Autodesk Fusion 360 part; units mm, degrees
sketch "Sketch1" plane through (0, 0, 0) normal (0, 1, 0) x (1, 0, 0)
  line L0 (0, 0) -> (82.5, 0)
  line L1 (82.5, 0) -> (82.5, -70)
  line L2 (82.5, -70) -> (0, -70)
  line L3 (0, -70) -> (0, 0)
  line L4 (2.54, -70) -> (2.54, -48.5)
  line L5 (2.54, -48.5) -> (0, -46.5)
  line L6 (2.54, 0) -> (2.54, -11.5)
  line L7 (2.54, -11.5) -> (0, -13.5)
  dimension "d1" = 82.5
  dimension "d2" = 70
  dimension "d3" = 33
  dimension "d4" = 11.5
  dimension "d5" = 2.54
  dimension "d6" = 2.54
  dimension "d7" = 21.5
  dimension "d8" = 2
extrude "Extrude1" add sketch "Sketch1" along normal blind 2 contours L0 L1 L2 L3 L4 L5 L6 L7
sketch "Sketch2" plane through (0, 2, 0) normal (0, 1, 0) x (-1, 0, 0)
  line L0 (-2.54, 0) -> (-2.54, 11.5)
  line L1 (-2.54, 11.5) -> (0, 13.5)
  line L2 (0, 13.5) -> (0, 46.5)
  line L3 (0, 46.5) -> (-2.54, 48.5)
  line L4 (-2.54, 48.5) -> (-2.54, 70)
  line L5 (-2.54, 70) -> (-82.5, 70)
  line L6 (-82.5, 70) -> (-82.5, 0)
  line L7 (-82.5, 0) -> (-2.54, 0)
  circle A0 centre (-2.54, 44.5) radius 1.6
  circle A1 centre (-54.14, 59.13) radius 1.6
  circle A2 centre (-55.54, 10.87) radius 1.6
  dimension "d11" = 3.2
  dimension "d12" = 2.54
  dimension "d13" = 33
  dimension "d14" = 3.2
  dimension "d15" = 3.2
  dimension "d17" = 10.87
  dimension "d20" = 53
  dimension "d21" = 51.6
  dimension "d22" = 48.26
extrude "Extrude2" cut sketch "Sketch2" against normal blind 2 contours A0 | A1 | A2
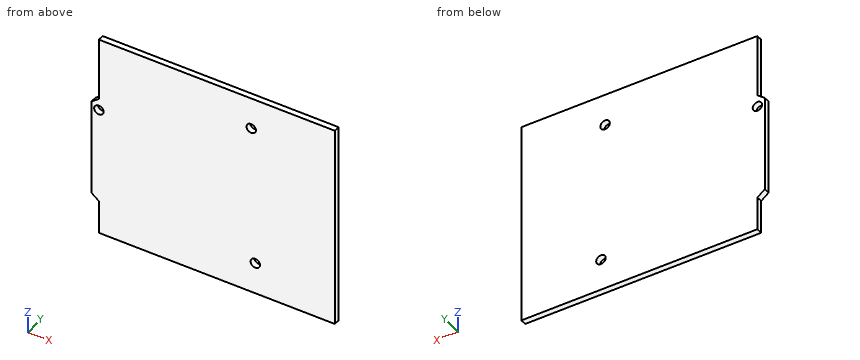
Check sheet for the modelled part. Datum: model origin and axes. Units: mm. Coordinates: 2 decimals unless noted, no trailing zeros. Order: outer loops, then holes, each group sorted by start corner. A loop starts at its lowest first (then second) coordinate and runs counter-clockwise, first axis right, second up. Notation, with made-up numbers: (78, 85.25) -> (135, 85.25) arc R24 ccw to (135, 124.25) -> close; hole circle Ø7 at (59, -10.75). An arc over 180 degrees is marked (long way). Write each question's results on one line, items separated by ' | '. Start each with the question number.
1) Material ranges on line 1 along Z through (x, y) = (55.54, 1.05); line 2 along Z through (x, y) = (54.14, 1); line 3 along X through (y, z) = (1.75, 55), recorded low to high.
2) Depth check by flat-ended pin: pin 1 (12 mm diameter, centred on x = 67, z = 37.5, fed in from -Y); pin 2 (1 mm diameter, centred on y = 1, z = 51, fed in from -X). Enter the tip coordinate at first touch or a pass-through.
3) Section check A-A (z = 44.5). Enter the section's corners in (x, y).
4) Section check B-B (y = 1.3). Enter the section's corners in (x, z), and give its area (3 significant figures).
Checked values:
1) line 1: 0 to 9.27, 12.47 to 58.36, 59.9 to 70 | line 2: 0 to 10.1, 11.64 to 57.53, 60.73 to 70 | line 3: 2.54 to 82.5
2) pin 1: y = 0 | pin 2: x = 2.54
3) outline: (0, 0) -> (0.94, 0) -> (0.94, 2) -> (0, 2) -> close; (4.14, 0) -> (82.5, 0) -> (82.5, 2) -> (4.14, 2) -> close
4) outline: (0, 13.5) -> (2.54, 11.5) -> (2.54, 0) -> (82.5, 0) -> (82.5, 70) -> (2.54, 70) -> (2.54, 48.5) -> (0, 46.5) -> close; hole circle Ø3.2 at (2.54, 44.5); hole circle Ø3.2 at (54.14, 59.13); hole circle Ø3.2 at (55.54, 10.87) | area: 5,660 mm²
